```python
from build123d import *

# Parameters (mm, degrees)
SKETCH_1_W                       = 40
SKETCH_1_H                       = 40
EXTRUDE_1_DEPTH                  = 100
SKETCH_2_R                       = 3.4
CUT_EXTRUDE_1_DEPTH              = 104.923048454
PATTERN_CIRCULAR_1_COUNT         = 4
FILLET_1_R                       = 2
SKETCH_4_W                       = 6.75
SKETCH_4_H                       = 6.75
CUT_EXTRUDE_2_DEPTH              = 104.923048454
FILLET_2_R                       = 1
FILLET_4_R                       = 2
PATTERN_CIRCULAR_2_COUNT         = 4
FILLET_2_OF_PATTERN_CIRCULAR_2_R = 1
FILLET_4_OF_PATTERN_CIRCULAR_2_R = 2


with BuildPart() as part:
    # Sketch 1 → Extrude 1 (new body)
    with BuildSketch(Plane.XY):
        Rectangle(SKETCH_1_W, SKETCH_1_H)
    extrude(amount=EXTRUDE_1_DEPTH)

    # Sketch 2 → Cut-Extrude 1 (cut, through all)
    with BuildSketch(Plane.XY.offset(100)):
        Polygon((-19.1, -4.1), (-18.2, -4.1), (-18.2, -10.25), (-12.15, -10.25), (-4.5, -2.6), (-4.5, 2.6), (-12.15, 10.25), (-18.2, 10.25), (-18.2, 4.1), (-19.1, 4.1), (-19.1, 5.1), (-20, 5.1), (-20, -5.1), (-19.1, -5.1), align=None)
        Circle(SKETCH_2_R)
    cut_extrude_1 = extrude(amount=-CUT_EXTRUDE_1_DEPTH, mode=Mode.SUBTRACT)

    # Pattern Circular 1: Cut-Extrude 1 ×4 about axis
    pattern_circular_1_axis = Axis((0, 0, 0), (0, 0, 1))
    for i in range(1, PATTERN_CIRCULAR_1_COUNT):
        add(cut_extrude_1.rotate(pattern_circular_1_axis, i * 360 / PATTERN_CIRCULAR_1_COUNT), mode=Mode.SUBTRACT)

    # Fillet 1
    fillet_1_edges = [part.edges().sort_by_distance(p)[0] for p in [
        (20, -20, 50),
        (-20, -20, 50),
        (-20, 20, 50),
        (20, 20, 50),
    ]]
    fillet(fillet_1_edges, radius=FILLET_1_R)

    # Sketch 4 → Cut-Extrude 2 (cut, symmetric)
    with BuildSketch(Plane.XY.offset(100)):
        with Locations((-15.125, 15.125)):
            Rectangle(SKETCH_4_W, SKETCH_4_H)
    cut_extrude_2 = extrude(amount=CUT_EXTRUDE_2_DEPTH, both=True, mode=Mode.SUBTRACT)

    # Fillet 2
    fillet_2_edges = [part.edges().sort_by_distance(p)[0] for p in [
        (-18.5, 11.75, 50),
        (-11.75, 18.5, 50),
        (-11.75, 11.75, 50),
    ]]
    fillet(fillet_2_edges, radius=FILLET_2_R)

    # Fillet 4
    fillet_4_edges = [part.edges().sort_by_distance(p)[0] for p in [
        (-18.5, 18.5, 50),
    ]]
    fillet(fillet_4_edges, radius=FILLET_4_R)

    # Pattern Circular 2: Cut-Extrude 2 ×4 about axis
    pattern_circular_2_axis = Axis((0, 0, 0), (0, 0, 1))
    for i in range(1, PATTERN_CIRCULAR_2_COUNT):
        add(cut_extrude_2.rotate(pattern_circular_2_axis, i * 360 / PATTERN_CIRCULAR_2_COUNT), mode=Mode.SUBTRACT)

    # Fillet 2 of Pattern Circular 2
    fillet_2_of_pattern_circular_2_edges = [part.edges().sort_by_distance(p)[0] for p in [
        (-11.75, -18.5, 50),
        (-18.5, -11.75, 50),
        (-11.75, -11.75, 50),
        (18.5, -11.75, 50),
        (11.75, -18.5, 50),
        (11.75, -11.75, 50),
        (11.75, 18.5, 50),
        (18.5, 11.75, 50),
        (11.75, 11.75, 50),
    ]]
    fillet(fillet_2_of_pattern_circular_2_edges, radius=FILLET_2_OF_PATTERN_CIRCULAR_2_R)

    # Fillet 4 of Pattern Circular 2
    fillet_4_of_pattern_circular_2_edges = [part.edges().sort_by_distance(p)[0] for p in [
        (-18.5, -18.5, 50),
        (18.5, -18.5, 50),
        (18.5, 18.5, 50),
    ]]
    fillet(fillet_4_of_pattern_circular_2_edges, radius=FILLET_4_OF_PATTERN_CIRCULAR_2_R)


solid = part.part
```
Can you work these out from the model? Positions are in its coordinate system, mm. A direction names the side the tool comes from. Coordinates: 2 decimals unless noted, no trailing zeros. Write each loop counter-clockwise with the first axis right and the second up, starting at its lowest first coordinate (ties: lowest second). Pieces come first, ordered by that corner, then holes. Notation, with made-up numbers: M 72,51.25 L 86,51.25 A27 cw 86,70.25 Z; hole C -31,80.25 d1. An arc over 180 degrees is marked long. Write item = value, one per line. Start each with the question number.
Q1. If we section it at B-B, the plane x = 0: Write out the boundary of the cut face in (y, z).
Q2. If I drill on L1, parallel to X at y = -16.5, z = 88; L2, parallel to X at y = 0, z = 72.5; L3, parallel to X at y = -5, z = 25, over which ranges is the centre line in solid material (lowest first)? Write a range as [from, to].
Q3. On a 3-axis mill with a long thin cutter (end or side, diameter ignored), from which of +Z, -Z, +X, -X, +Y, -Y can I reach the whole of each face in a straight line? I mean faces 5 (the face through (-19.43, -19.4, 50.7)), 6 (the face through (8.4, 6.5, 50.7)). Say none if no direction works.
Q4. If we section it at D-D, the plane x = 8.5: Write out the boundary of the cut face in (y, z).
Q5. If we section it at A-A, the plane y = 8: Write out the boundary of the cut face in (x, z), then the cut area to 3 significant figures.
Q6. Thinking about a two-plate mould opening in Y: for faces 1 (the face through (11, 20, 49)), 2 (the face through (-20, 11, 49)), 3 (the face through (-4.5, 0, 51)), 4 (the face through (-10.25, -15, 51)), which applies, released by +Y, released by -Y, zero draft, split by the parting line, or undercut?
Q7. I'm going to push flat-ended pins straight in: pin 1 (5.5 mm diameter, centred on y = 0, z = 57.5, fed in from +X); pin 2 (1.5 mm diameter, centred on x = 9, y = 13.5, fed in from -Z); pin 3 (3 mm diameter, centred on x = 0, z = 11, fed in from -Y); pin 4 (0.7 mm diameter, centred on y = -19.5, z = 72, fed in from -X). Where does each tip first touch, or does it pass through?
Check sheet entries:
q1.outline = M -4.5,0 L -3.4,0 L -3.4,100 L -4.5,100 Z; M 3.4,0 L 4.5,0 L 4.5,100 L 3.4,100 Z
q2.L1 = [-20, -18.5], [-11.75, -10.25], [10.25, 11.75], [18.5, 20]
q2.L2 = [-4.5, -3.4], [3.4, 4.5]
q2.L3 = [-19.1, -18.2], [-6.9, -3.1], [3.1, 6.9], [18.2, 19.1]
q3.face_5 = +Z, -Z, -X, -Y
q3.face_6 = +Z, -Z
q4.outline = M -20,0 L -18.2,0 L -18.2,100 L -20,100 Z; M -10.4,0 L -6.6,0 L -6.6,100 L -10.4,100 Z; M 6.6,0 L 10.4,0 L 10.4,100 L 6.6,100 Z; M 18.2,0 L 20,0 L 20,100 L 18.2,100 Z
q5.outline = M -20,0 L -18.2,0 L -18.2,100 L -20,100 Z; M -9.9,0 L -6.1,0 L -6.1,100 L -9.9,100 Z; M 6.1,0 L 9.9,0 L 9.9,100 L 6.1,100 Z; M 18.2,0 L 20,0 L 20,100 L 18.2,100 Z
q5.area = 1,120 mm²
q6.face_1 = released by +Y
q6.face_2 = zero draft
q6.face_3 = undercut
q6.face_4 = undercut
q7.pin_1 = 4.65
q7.pin_2 = through
q7.pin_3 = -4.5
q7.pin_4 = -19.64
